Geometry: final body of the model. Coordinates: model frame, mm. Face numbers are marked on the shaded views. A direction names the side the tool comes from. Give positions to 0.01 mm unless a question says otherwise; leave off trailing zeros. Loops run counter-clockwise (first coordinate to the right, second up) from the corner with the lowest first, then second, coordinate; pieces in that order, holes last. Notation, with made-up numbers: M 89.5,14 L 145.5,14 A22 ccw 145.5,27 Z; hole C -36,49 d10. An arc over 180 degrees is marked long. One line per question, with ' | ' between items. Start each with the question number.
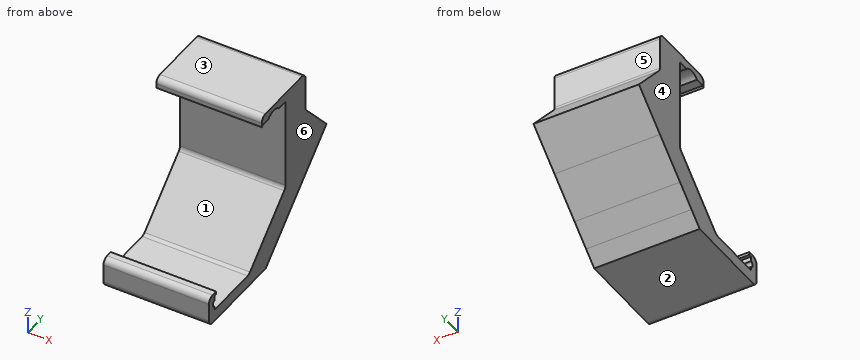
from build123d import *

# Parameters (mm, degrees)
F1_DEPTH = 35
F3_DEPTH = 35
F5_DEPTH = 35
F7_DEPTH = 35.001
F8_R     = 2


with BuildPart() as f1:
    # F0 (on Right) → F1 (new body)
    with BuildSketch(Plane.YZ):
        Polygon((19, 0), (0, 0), (0, 5), (1, 5), (1, 6), (-3, 6), (-3, -4), (28.1972419471, -4), (32.6792613945, 0), align=None)
        Polygon((39, 17.8490970284), (19, 0), (32.6792613945, 0), (39, 5.6409738331), align=None)
        Polygon((39, 49), (39, 17.8490970284), (39, 5.6409738331), (50, 15.4579771987), (50, 38.7150122165), (50, 52), (26, 52), (26, 49), align=None)
        Polygon((50, 38.7150122165), (50, 15.4579771987), (61.5536515036, 25.7690895346), align=None)
    extrude(amount=F1_DEPTH)

    # F2 (on face) → F3 (join)
    with BuildSketch(Plane.YZ):
        Polygon((26.4567731472, 49), (26, 49), (26, 48.5158836246), align=None)
    extrude(amount=F3_DEPTH)

    # F4 (on Right) → F5 (cut, through all)
    with BuildSketch(Plane.YZ):
        with BuildLine():
            Line((29.6401511878, 49), (35.453248769, 49))
            ThreePointArc((35.453248769, 49), (32.5466999784, 50.1759769875), (29.6401511878, 49))
        make_face()
    extrude(amount=F5_DEPTH, mode=Mode.SUBTRACT)

    # F6 (on face) → F7 (cut, through all)
    with BuildSketch(Plane.YZ):
        with BuildLine():
            Line((0, 1.3031382114), (0, 3.3907820471))
            ThreePointArc((0, 3.3907820471), (-0.8807520402, 2.3469601292), (0, 1.3031382114))
        make_face()
    extrude(amount=F7_DEPTH, mode=Mode.SUBTRACT)

    # F8
    f8_edges = [f1.edges().sort_by_distance(p)[0] for p in [
        (17.5, 50, 52),
        (17.5, -3, -4),
        (17.5, -3, 6),
        (17.5, 26, 52),
        (17.5, 39, 17.849097),
        (17.5, 19, 0),
        (17.5, 50, 38.715012),
    ]]
    fillet(f8_edges, radius=F8_R)


solid = f1.part
Q1. Set-up query: the marked faces 5 and 6. Return all of +Z, -Z, +X, -X, +Y, -Y with unobstructed straight access to the full face (end or side cutting, diameter ignored); none if empty.
Q2. Section C-C, the plane z = 22. Output: boundary loops of the cut face in (x, y), plus the area to 3 significant figures.
Q3. Material intervals for L1, parallel to Y at x = 20, z = 43.5; L2, parallel to Z at x = 19, y = 6.5; L3, parallel to Z at x = 10.5, y = 31, sorted ascending.
Q4. Draft query along Z for the marked faces 1, 2, 3 and 4. Return one class per face: released by +Z, released by -Z, zero draft, split by the parting line, or undercut.
Q5. Section B-B, the plane y = 10.5. Output: boundary loops of the cut face in (x, z).
Q6. Contact query for flat-ended pins moving along their axis: pin 1 (5 mm diameter, centred on x = 16, z = 16.5, fed in from +Y); pin 2 (12 mm diameter, centred on x = 12, z = 37, fed in from -Y); pin 3 (3 mm diameter, centred on x = 20.5, y = 38, fed in from -Z); pin 4 (2.5 mm diameter, centred on x = 26, y = 28.5, fed in from -Z). Output: stop coordinate, or through.
Q7. Section A-A, the plane x = 31.5. Output: boundary loops of the cut face in (y, z).
Model answer:
1) face 5: +Z, +X, -X, +Y | face 6: +Z, -Z, +X, +Y, -Y
2) outline: M 0,39 L 35,39 L 35,57.33 L 0,57.33 Z | area: 642 mm^2
3) L1: y = 39 to 50 | L2: z = -4 to 0 | L3: z = -1.5 to 10.71, 49.88 to 52
4) face 1: undercut | face 2: released by -Z | face 3: released by +Z | face 4: zero draft
5) outline: M 0,-4 L 35,-4 L 35,0 L 0,0 Z
6) pin 1: stops at y = 53.97 | pin 2: stops at y = 39 | pin 3: stops at z = 3.41 | pin 4: stops at z = -4
7) outline: M -3,-2 A2 ccw -1,-4 L 28.2,-4 L 61.55,25.77 L 50.51,38.15 A2 cw 50,39.48 L 50,50 A2 ccw 48,52 L 28,52 A2 ccw 26,50 L 26,48.52 L 26.46,49 L 29.64,49 A4.18 cw 35.45,49 L 39,49 L 39,18.74 A2 cw 38.33,17.25 L 19.57,0.51 A2 cw 18.24,0 L 0,0 L 0,1.3 A1.06 cw 0,3.39 L 0,5 L 1,5 L 1,6 L -1,6 A2 ccw -3,4 Z
